For this review, take the finished solid that the model builds, in its own axes (mm). A direction names the side the tool comes from. Coordinates: 2 decimals unless noted, no trailing zeros. Order: outer loops, then holes, each group sorted by start corner. A loop starts at its lowest first (then second) coordinate and runs counter-clockwise, first axis right, second up. Notation, with made-up numbers: (31, -21.75) -> (40, -21.75) arc R34 ccw to (40, 15.25) -> close; hole circle Ø6 at (31, 57.25). An arc over 180 degrees is marked (long way). Return JSON: item names as keys, results as strings. Group by question number.
Item 1: Machinability: for faces 1 (the flat face through (-1, 50.35, 21)), 2 (the flat face through (-1, 24.85, 16)), which of the approach directions +Z, -Z, +X, -X, +Y, -Y give a long, thin tool a straight path to every point of the face, cutting with its end or side? Answer none if there is none.
Item 2: Insertion check: pin 1 (6 mm diameter, centred on x = -36, y = 2, fed in from +Z). The pin has a flat end and moves straight along its axis. Give the tip position at first contact, or say it passes through.
Item 3: Draft analysis for pull direction X (two halves, no side actions). For faces 3 (the flat face through (-1, 1, 0)), 4 (the flat face through (-1, 37, 2.6)), 5 (the flat face through (-51.35, -1, 21)), state which applies: +X half, -X half, draft (parallel to the pull), parting line (faces both ways), or undercut.
Item 4: Take a section at B-B (x = -31). Write out the cut boundary in (y, z), then the cut area to 3 significant figures.
Item 5: Take a section at A-A (z = 36). Write out the cut boundary in (x, y).
Item 6: Take a section at C-C (y = -7). Write out the cut boundary in (x, z), then the cut area to 3 significant figures.
Item 7: For line 1 along Y through (x, z) = (-23, 23.5); line 2 along X through (y, z) = (41.5, 34.5); line 3 along Y through (x, z) = (19, 38), list the stretches that pass through material, from the lowest coordinate up.
Item 8: Take a section at D-D (z = 23). Write out the cut boundary in (x, y).
```python
from build123d import *

# Parameters (mm, degrees)
F0_W     = 99.7
F0_H     = 24
F1_DEPTH = 2.6
F0_H_2   = 73.7
F2_DEPTH = 30
F0_W_2   = 102.7
F0_H_3   = 100.7
F3_DEPTH = 42


with BuildPart() as f1:
    # F0 (on Top) → F1 (new body)
    with BuildSketch(Plane.XY):
        with Locations((0, 36.85)):
            Rectangle(F0_W, F0_H)
    extrude(amount=F1_DEPTH)

    # F0 (on Top) → F2 (join)
    with BuildSketch(Plane.XY):
        with Locations((0, -12)):
            Rectangle(F0_W, F0_H_2)
    extrude(amount=F2_DEPTH)

    # F0 (on Top) → F3 (join)
    with BuildSketch(Plane.XY):
        Rectangle(F0_W_2, F0_H_3)
        Polygon((-49.85, 24.85), (-49.85, 48.85), (49.85, 48.85), (49.85, 24.85), (49.85, -48.85), (-49.85, -48.85), align=None, mode=Mode.SUBTRACT)
    extrude(amount=F3_DEPTH)


solid = f1.part
```
Findings below:
{
 "1": {"face 1": "+Z, -Z, +X, -X, +Y", "face 2": "+Z"},
 "2": {"pin 1": "stops at z = 30"},
 "3": {"face 3": "draft", "face 4": "undercut", "face 5": "-X half"},
 "4": {"outline": "(-50.35, 0) -> (50.35, 0) -> (50.35, 42) -> (48.85, 42) -> (48.85, 2.6) -> (24.85, 2.6) -> (24.85, 30) -> (-48.85, 30) -> (-48.85, 42) -> (-50.35, 42) -> close", "area": "2,400 mm2"},
 "5": {"outline": "(-51.35, -50.35) -> (51.35, -50.35) -> (51.35, 50.35) -> (-51.35, 50.35) -> close; hole (-49.85, -48.85) -> (49.85, -48.85) -> (49.85, 48.85) -> (-49.85, 48.85) -> close"},
 "6": {"outline": "(-51.35, 0) -> (51.35, 0) -> (51.35, 42) -> (49.85, 42) -> (49.85, 30) -> (-49.85, 30) -> (-49.85, 42) -> (-51.35, 42) -> close", "area": "3,120 mm2"},
 "7": {"line 1": "y = -50.35 to 24.85, 48.85 to 50.35", "line 2": "x = -51.35 to -49.85, 49.85 to 51.35", "line 3": "y = -50.35 to -48.85, 48.85 to 50.35"},
 "8": {"outline": "(-51.35, -50.35) -> (51.35, -50.35) -> (51.35, 50.35) -> (-51.35, 50.35) -> close; hole (-49.85, 24.85) -> (49.85, 24.85) -> (49.85, 48.85) -> (-49.85, 48.85) -> close"}
}
